```python
from build123d import *

# Parameters (mm, degrees)
SKETCH1_R           = 4
BOSS_EXTRUDE1_DEPTH = 3
BOSS_EXTRUDE2_DEPTH = 3
FILLET1_R           = 3


with BuildPart() as part:
    # Sketch1 → Boss-Extrude1 (new body)
    with BuildSketch(Plane.XY):
        with BuildLine():
            Line((-5, 5.590169944), (-5, 18))
            Line((-5, 18), (5, 18))
            Line((5, 18), (5, 5.590169944))
            ThreePointArc((5, 5.590169944), (0, -7.5), (-5, 5.590169944))
        make_face()
        Circle(SKETCH1_R, mode=Mode.SUBTRACT)
    extrude(amount=BOSS_EXTRUDE1_DEPTH)

    # Sketch2 → Boss-Extrude2 (add)
    with BuildSketch(Plane(origin=(0, 0, 0), x_dir=(-1, 0, 0), z_dir=(0, 0, -1))):
        with BuildLine():
            Line((-4.283653157, -6.156323223), (-14.506679921, 0.956997388))
            Line((-14.506679921, 0.956997388), (-3.437791444, 6.665702513))
            ThreePointArc((-3.437791444, 6.665702513), (-7.483733204, 0.493697605), (-4.283653157, -6.156323223))
        make_face()
        with BuildLine():
            Line((4.283653157, -6.156323223), (14.506679921, 0.956997388))
            Line((14.506679921, 0.956997388), (3.437791444, 6.665702513))
            ThreePointArc((3.437791444, 6.665702513), (7.483733204, 0.493697605), (4.283653157, -6.156323223))
        make_face()
    extrude(amount=-BOSS_EXTRUDE2_DEPTH)

    # Fillet1
    fillet1_edges = [part.edges().sort_by_distance(p)[0] for p in [
        (14.506679921, 0.956997388, 1.5),
        (-14.506679921, 0.956997388, 1.5),
    ]]
    fillet(fillet1_edges, radius=FILLET1_R)


solid = part.part
```
Verification items for the finished model (mm, model axes). A direction names the side the tool comes from. Give positions to 0.01 mm unless a question says otherwise; leave off trailing zeros. Order: outer loops, then holes, each group sorted by start corner. A loop starts at its lowest first (then second) coordinate and runs counter-clockwise, first axis right, second up. Notation, with made-up numbers: (20.5, -7) - (54.5, -7) arc R22 ccw to (54.5, 12) - close; hole circle Ø8 at (1, 76.5). An arc over 180 degrees is marked (long way). Answer as CSV lines item,"result". Start each with the question number.
Item 1: Access from +Z, -Z, +X, -X, +Y, -Y to the whole of each face (thin tool, end or side, straight path). Record for faces 5 (the face through (5, 12, 1)), 6 (the face through (-5, 12, 1)), 7 (the face through (11.7, 0.7, 1.5)).
Item 2: Gauge pin test, flat end, axial feed: pin 1 (1 mm diameter, centred on x = 6.5, z = 1.5, fed in from +Y). Record the tip position at first contact, or that the pin passes through.
Item 3: Section check B-B, the plane z = 1.4. Record the boundary of the cut face in (x, y).
Item 4: Material ranges on L1, parallel to Y at x = 0, z = 2.1; L2, parallel to X at y = 15, z = 2.7; L3, parallel to X at y = -1, z = 2.05, recorded low to high.
Item 5: Section check D-D, the plane x = -8. Record the boundary of the cut face in (y, z), plus the area to 3 significant figures.
Item 6: Section check C-C, the plane y = 0. Record the boundary of the cut face in (x, z).
Item 7: Section check A-A, the plane x = 0. Record the boundary of the cut face in (y, z).
Item 8: Mould release check, pull along X, two halves, no side actions. Record for faces 1 (the face through (-0.867, -3.905, 1.479)), 2 (the face through (0, 5, 0)), 3 (the face through (7.31, -4.05, 1.48)), 4 (the face through (-7.31, -4.05, 1.48)): released by +X, released by -X, zero draft, split by the parting line, or undercut.
Filled in:
1,face 5,"+Z, -Z, +X, +Y"
1,face 6,"+Z, -Z, -X, +Y"
1,face 7,"+Z, -Z, +X"
2,pin 1,"y = 5.34"
3,outline,"(-10.42, -1.89) - (-4.28, -6.16) arc R7.5 ccw to (4.28, -6.16) - (10.42, -1.89) arc R3 ccw to (10.08, 3.24) - (5, 5.86) - (5, 18) - (-5, 18) - (-5, 5.86) - (-10.08, 3.24) arc R3 ccw to start; hole circle Ø8 at (0, 0)"
4,L1,"-7.5 to -4, 4 to 18"
4,L2,"-5 to 5"
4,L3,"-11.26 to -3.87, 3.87 to 11.26"
5,outline,"(-3.57, 0) - (4.31, 0) - (4.31, 3) - (-3.57, 3) - close"
5,area,"23.6 mm^2"
6,outline,"(-11.65, 0) - (-4, 0) - (-4, 3) - (-11.65, 3) - close; (4, 0) - (11.65, 0) - (11.65, 3) - (4, 3) - close"
7,outline,"(-7.5, 0) - (-4, 0) - (-4, 3) - (-7.5, 3) - close; (4, 0) - (18, 0) - (18, 3) - (4, 3) - close"
8,face 1,"undercut"
8,face 2,"zero draft"
8,face 3,"released by +X"
8,face 4,"released by -X"
